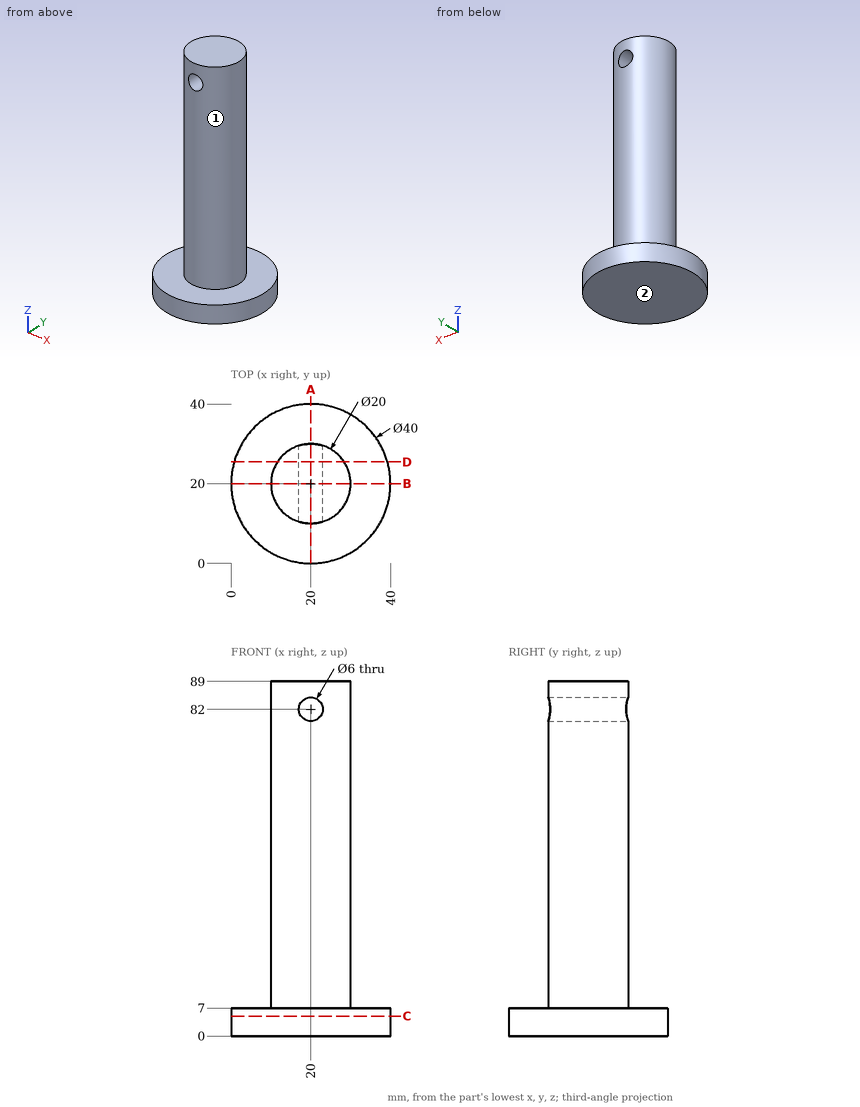
Verification items for this drawing (mm, ordinates from the low corner). A direction names the side the tool comes from. Coordinates: 2 decimals unless noted, no trailing zeros. Loops run counter-clockwise (first coordinate to the right, second up) from the corner with the lowest first, then second, coordinate; pieces in that order, holes last. Notation, with made-up numbers: (-29, -7.5) - (-10, -7.5) arc R19 cw to (-10, 15.5) - close; hole circle Ø2 at (69, 21). An arc over 180 degrees is marked (long way). One line per item, written item: value. Start each with the question number.
(1) Cross-section at B-B on y = 20. Enter the section's corners in (x, z), plus the area to 3 significant figures.
(2) Tool access check on the marked faces 1 and 2. Record the directions out of +Z, -Z, +X, -X, +Y, -Y that give a thin tool (end or side, any length) a straight path to the whole face; none if there is none.
(3) Cross-section at D-D on y = 25.5. Enter the section's corners in (x, z), plus the area to 3 significant figures.
(4) Depth check by flat-ended pin: P1, Ø4, axis at x = 6, z = 9.5, coming from the +Y side; P2, Ø1, axis at x = 12.5, y = 29, coming from the +Z side; P3, Ø12, axis at x = 25, z = 76, coming from the -Y side; P4, Ø8, axis at x = 22, z = 43.5, coming from the +Y side. Enter the tip coordinate at first touch or a pass-through.
(5) Material ranges on line 1 (Z direction, x = 20, y = 15); line 2 (Z direction, x = 8.5, y = 34); line 3 (X direction, y = 20.5, z = 82), recorded low to high. Write a range as [from, to].
(6) Cross-section at A-A on x = 20. Enter the section's corners in (y, z).
(7) Cross-section at C-C on z = 5. Enter the section's corners in (x, y).
Results below:
1. outline: (0, 0) - (40, 0) - (40, 7) - (30, 7) - (30, 89) - (10, 89) - (10, 7) - (0, 7) - close; hole circle Ø6 at (20, 82)
1. area: 1,890 mm2
2. face 1: +Z
2. face 2: -Z, +X, -X, +Y, -Y
3. outline: (0.77, 0) - (39.23, 0) - (39.23, 7) - (28.35, 7) - (28.35, 89) - (11.65, 89) - (11.65, 7) - (0.77, 7) - close; hole circle Ø6 at (20, 82)
3. area: 1,610 mm2
4. P1: passes through
4. P2: stops at z = 7
4. P3: stops at y = 10
4. P4: stops at y = 30
5. line 1: z = [0, 79], [85, 89]
5. line 2: z = [0, 7]
5. line 3: x = [10.01, 17], [23, 29.99]
6. outline: (0, 0) - (40, 0) - (40, 7) - (30, 7) - (30, 79) - (10, 79) - (10, 7) - (0, 7) - close; (10, 85) - (30, 85) - (30, 89) - (10, 89) - close
7. outline: circle Ø40 at (20, 20)
